```python
from build123d import *

# Parameters (mm, degrees)
SKETCH1_R           = 2.05
BOSS_EXTRUDE1_DEPTH = 2
LPATTERN1_COUNT     = 20
LPATTERN1_PITCH     = 8


with BuildPart() as part:
    # Sketch1 → Boss-Extrude1 (new body)
    with BuildSketch(Plane.XY):
        Polygon((1.656854249, 4), (-1.656854249, 4), (-4, 1.656854249), (-4, -1.656854249), (-1.656854249, -4), (1.656854249, -4), (4, -1.656854249), (4, 1.656854249), align=None)
        Circle(SKETCH1_R, mode=Mode.SUBTRACT)
    boss_extrude1 = extrude(amount=BOSS_EXTRUDE1_DEPTH)

    # LPattern1: Boss-Extrude1 ×20
    with Locations(*[(i * LPATTERN1_PITCH, 0, 0) for i in range(1, LPATTERN1_COUNT)]):
        add(boss_extrude1)


solid = part.part
```
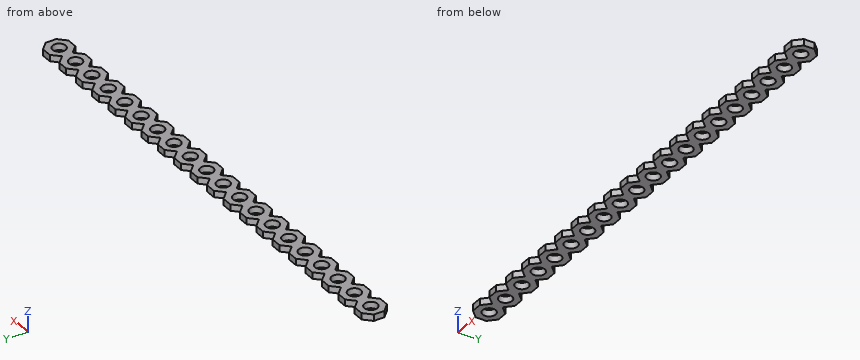
Part model, mm, in its own coordinate system. Give positions to 0.01 mm unless a question says otherwise; leave off trailing zeros. Write each loop counter-clockwise with the first axis right and the second up, starting at its lowest first coordinate (ties: lowest second). Pieces come first, ordered by that corner, then holes. Notation, with made-up numbers: (-9.75, 68.5) -> (45.25, 68.5) arc R23 cw to (45.25, 89.5) -> close; hole circle Ø1 at (68.25, -30.5). An arc over 180 degrees is marked (long way). Put each result on its own line as item: value. Start each with the question number.
Item 1: Cut at B-B (z = 1.45). State how many separate pieces and enclosed holes the cut face has, then the cut area to 3 significant figures.
Item 2: Pin check, flat tips, straight feed: pin 1 Ø3.5 at (x, y) = (32, 0) entering from +Z; pin 2 Ø1 at (x, z) = (76, 0.5) entering from -Y; pin 3 Ø4.5 at (x, y) = (24, 0) entering from +Z. Stop position of each tip, or through.
Item 3: Cut at A-A (x = 96). List the corners of the cut face in (y, z), then the cut area to 3 significant figures.
Item 4: Wall check: L1, parallel to Y at x = 56, z = 1.8; L2, parallel to Y at x = 44, z = 1.5; L3, parallel to Y at x = 77.5, z = 0.7. Give the ranges that are in metal, low to high. Write a range as [from, to].
Answer list:
1. separate pieces: 1
1. enclosed holes: 20
1. area: 796 mm2
2. pin 1: passes through
2. pin 2: stops at y = -2.16
2. pin 3: stops at z = 2
3. outline: (-4, 0) -> (-2.05, 0) -> (-2.05, 2) -> (-4, 2) -> close; (2.05, 0) -> (4, 0) -> (4, 2) -> (2.05, 2) -> close
3. area: 7.80 mm2
4. L1: y = [-4, -2.05], [2.05, 4]
4. L2: y = [-1.66, 1.66]
4. L3: y = [-3.16, 3.16]
